```python
from build123d import *

# Parameters (mm, degrees)
F0_W           = 32
F0_H           = 5
F1_DEPTH       = 25
F3_D           = 4
F3_CSINK_D     = 10
F3_CSINK_ANGLE = 90
F4_R           = 3.5


with BuildPart() as f1:
    # F0 (on Top) → F1 (new body)
    with BuildSketch(Plane.XY):
        with Locations((2.365528, -44.752212)):
            Rectangle(F0_W, F0_H)
        Polygon((-18.634472, -47.252212), (-13.634472, -47.252212), (-13.634472, -42.252212), (-13.634472, 27.747788), (-18.634472, 27.747788), align=None)
        Polygon((18.365528, -42.252212), (18.365528, -47.252212), (23.365528, -47.252212), (23.365528, 107.747788), (18.365528, 107.747788), align=None)
    extrude(amount=F1_DEPTH)

    # F3 (through all)
    with Locations(Plane(origin=(18.365528, 0, 0), x_dir=(0, -1, 0), z_dir=(-1, 0, 0))):
        with Locations((-97.990669, 12.5)):
            CounterSinkHole(F3_D / 2, F3_CSINK_D / 2, counter_sink_angle=F3_CSINK_ANGLE)

    # F4
    f4_edges = [f1.edges().sort_by_distance(p)[0] for p in [
        (-16.134472, 27.747788, 0),
        (-16.134472, 27.747788, 25),
        (20.865528, 107.747788, 0),
        (20.865528, 107.747788, 25),
        (-18.634472, 27.747788, 12.5),
        (-18.634472, -9.752212, 25),
        (-18.634472, -9.752212, 0),
        (-18.634472, -47.252212, 12.5),
        (2.365528, -47.252212, 25),
        (2.365528, -47.252212, 0),
        (18.365528, 107.747788, 12.5),
    ]]
    fillet(f4_edges, radius=F4_R)


solid = f1.part
```
For this review, take the finished solid that the model builds, in its own axes (mm). A direction names the side the tool comes from. Coordinates: 2 decimals unless noted, no trailing zeros. Write each loop counter-clockwise with the first axis right and the second up, starting at its lowest first coordinate (ties: lowest second). Pieces come first, ordered by that corner, then holes. Notation, with made-up numbers: (-31, -6.5) - (11, -6.5) arc R8 cw to (11, 6.5) - close; hole circle Ø7 at (63, 5). An arc over 180 degrees is marked (long way). Put each result on its own line as item: value.
1. Mouldability with a two-part tool opening along X and no side actions: class faces 1 (the cylindrical face through (-17.582, -10.228, 24.002)), 2 (the flat face through (18.366, 32, 12)), 3 (the cylindrical face through (4.4, -46.3, 1.1)) as released by +X, released by -X, zero draft, split by the parting line, or undercut.
Values found:
face 1: released by -X
face 2: undercut
face 3: zero draft
2. For pin 1 (1.2 mm diameter, centred on x = -14.5, z = 15.5, fed in from +Y); pin 2 (7.5 mm diameter, centred on y = 65, z = 18.5, fed in from -X), all flat-tipped, find the tip position at first contact; note any pin that passes through.
Values found:
pin 1: y = 27.75
pin 2: x = 18.37
3. Add section B-B, the plane z = 12.5. Give the boundary of the cut face in (x, y), then the cut area to 3 significant figures.
Values found:
outline: (-18.63, -43.75) arc R3.5 ccw to (-15.13, -47.25) - (23.37, -47.25) - (23.37, 95.99) - (21.37, 95.99) - (18.37, 92.99) - (18.37, -42.25) - (-13.63, -42.25) - (-13.63, 27.75) - (-15.13, 27.75) arc R3.5 ccw to (-18.63, 24.25) - close; (18.37, 102.99) - (21.37, 99.99) - (23.37, 99.99) - (23.37, 107.75) - (21.87, 107.75) arc R3.5 ccw to (18.37, 104.25) - close
area: 1,270 mm²
4. Add section D-D, the plane y = 33.5. Give the boundary of the cut face in (x, z), then the cut area to 3 significant figures.
Values found:
outline: (18.37, 0) - (23.37, 0) - (23.37, 25) - (18.37, 25) - close
area: 125 mm²
5. Add section A-A, the plane y = -20. Give the boundary of the cut face in (x, z).
Values found:
outline: (-18.63, 3.5) arc R3.5 ccw to (-15.13, 0) - (-13.63, 0) - (-13.63, 25) - (-15.13, 25) arc R3.5 ccw to (-18.63, 21.5) - close; (18.37, 0) - (23.37, 0) - (23.37, 25) - (18.37, 25) - close
6. Machinability: for faces 4 (the cylindrical face through (-14.4, 26.7, 24)), 5 (the cylindrical face through (-14.39, 26.75, 1.05)), 6 (the flat face through (-13.634, -8, 12)), which of the approach directions +Z, -Z, +X, -X, +Y, -Y give a long, thin tool a straight path to every point of the face, cutting with its end or side? Answer none if there is none.
Values found:
face 4: +Z, -X, +Y
face 5: -Z, -X, +Y
face 6: +Z, -Z, +Y
7. Wall thickness on probe 1 along X at (y, z) = (-13.5, 6.5); probe 2 along Y at (x, z) = (22.7, 12.5); probe 3 along Y at (x, z) = (0, 14): over which ranges is each line inside the solid? List them lowest first.
Values found:
probe 1: -18.63 to -13.63, 18.37 to 23.37
probe 2: -47.25 to 95.99, 99.99 to 107.75
probe 3: -47.25 to -42.25
8. Add section C-C, the plane x = 7. Give the boundary of the cut face in (y, z), then the cut area to 3 significant figures.
Values found:
outline: (-47.25, 3.5) arc R3.5 ccw to (-43.75, 0) - (-42.25, 0) - (-42.25, 25) - (-43.75, 25) arc R3.5 ccw to (-47.25, 21.5) - close
area: 120 mm²
